Autodesk Inventor part; units mm, degrees
ref_plane "YZ Plane" through (0, 0, 0) normal (1, 0, 0) x (0, 1, 0)
ref_plane "XZ Plane" through (0, 0, 0) normal (0, 1, 0) x (-1, 0, 0)
ref_plane "XY Plane" through (0, 0, 0) normal (0, 0, 1) x (1, 0, 0)
sketch "Skizze1" plane through (0, 0, 0) normal (0, 0, 1) x (1, 0, 0)
  circle A0 centre (0, 0) radius 3.25
  circle A1 centre (12, 0) radius 2
  line L0 (0, 0) -> (12, 0) construction
  line L1 (12.1001, 1.9975) -> (2.0767, 2.5)
  line L2 (2.0767, -2.5) -> (12.1001, -1.9975)
  dimension "d0" = 6.5
  dimension "d1" = 12
  dimension "d2" = 4
  dimension "d3" = 2.5
  dimension "d4" = 2.5
extrude "Extrusion1" add sketch "Skizze1" along normal blind 1
sketch "Skizze2" plane through (0, 0, 0) normal (0, 0, -1) x (-1, 0, 0)
  line L0 (-2.0767, -2.5) -> (-12.1001, -1.9975)
  circle A0 centre (0, 0) radius 3.25
extrude "Extrusion2" add sketch "Skizze2" along normal blind 3
sketch "Skizze3" plane through (0, 0, 1) normal (0, 0, 1) x (1, 0, 0)
  arc A0 (12.1001, -1.9975) -> (12.1001, 1.9975) centre (12, 0) ccw
  circle A1 centre (12, 0) radius 0.5
  circle A2 centre (10, 0) radius 1
  point P0 (0, 0)
  dimension "d9" = 2
  dimension "d10" = 1
  dimension "d11" = 2
extrude "Extrusion3" cut sketch "Skizze3" against normal blind 3.25
sketch "Skizze4" plane through (0, 0, 1) normal (0, 0, 1) x (1, 0, 0)
  circle A0 centre (0, 0) radius 1.5
  dimension "d14" = 3
extrude "Extrusion4" cut sketch "Skizze4" against normal blind 6.25
properties part number "P_Servo_SIMPROP_lever"
Read the model definition and answer for the solid it produces. Units are mm, in the model's axes. Give positions to 0.01 mm unless a question says otherwise; leave off trailing zeros. Write each loop counter-clockwise with the first axis right and the second up, starting at its lowest first coordinate (ties: lowest second). Pieces come first, ordered by that corner, then holes. Notation, with made-up numbers: (78, 3) - (92, 3) arc R12 ccw to (92, 25) - close; hole circle Ø6 at (19.5, 16). An arc over 180 degrees is marked (long way). Write item = value, one per line. Start each with the question number.
Item 1: The mould has two halves that part along X. Classify faces 1 (the flat face through (7.159, 2.245, 0.493)), 2 (the cylindrical face through (11.5, 0, 0.5)), 3 (the flat face through (5, 0, 1)): +X half, -X half, draft (parallel to the pull), parting line (faces both ways), or undercut.
Item 2: Find section B-B (z = -0.65). Give the vertices of the cut face in (x, y), then the cut area to 3 significant figures.
Item 3: Each of these flat-tipped pins is pushed along its axis until it touches: P1, Ø2, axis at x = 8, y = -2, coming from the -Z side; P2, Ø1, axis at x = 2, z = -0.5, coming from the +Y side; P3, Ø1.2, axis at x = 10, y = 0, coming from the +Z side. Where does it stop, or does it pass through?
Item 4: Find the intervals of material crossed by probe 1 along X at (y, z) = (0.75, 0.2); probe 2 along Y at (x, z) = (0, -0.3); probe 3 along Y at (x, z) = (9.25, 0.8), in increasing order. Write a range as [from, to].
Item 5: Find section D-D (x = 13.25). Give the vertices of the cut face in (y, z).
Item 6: Find section A-A (x = 10). Give the vertices of the cut face in (y, z).
Response:
q1.face_1 = +X half
q1.face_2 = undercut
q1.face_3 = draft
q2.outline = circle Ø6.5 at (0, 0); hole circle Ø3 at (0, 0)
q2.area = 26.1 mm²
q3.P1 = 0
q3.P2 = 2.88
q3.P3 = through
q4.probe_1 = [-3.16, -1.3], [1.3, 9.34], [10.66, 13.85]
q4.probe_2 = [-3.25, -1.5], [1.5, 3.25]
q4.probe_3 = [-2.14, -0.66], [0.66, 2.14]
q5.outline = (-1.56, 0) - (1.56, 0) - (1.56, 1) - (-1.56, 1) - close
q6.outline = (-2.1, 0) - (-1, 0) - (-1, 1) - (-2.1, 1) - close; (1, 0) - (2.1, 0) - (2.1, 1) - (1, 1) - close
